Work out the finished part from the listing and answer in its coordinate system (mm). Face numbers are marked on the shaded views. A direction names the side the tool comes from. Give positions to 0.01 mm unless a question says otherwise; leave off trailing zeros. Loops run counter-clockwise (first coordinate to the right, second up) from the corner with the lowest first, then second, coordinate; pieces in that order, holes last. Notation, with made-up numbers: (39.25, 16) -> (71.25, 16) arc R22 cw to (71.25, 52) -> close; hole circle Ø9 at (19, -23). An arc over 180 degrees is marked (long way). Answer as CSV lines item,"result". Start each with the question number.
1. Find the intervals of material crossed by line 1 along X through (y, z) = (2.2, 8); line 2 along X through (y, z) = (4.35, 5); line 3 along Z through (x, y) = (31.5, 0.7), in increasing order.
2. Find section D-D, the plane z = -11. Give the vertices of the cut face in (x, y), and give its area (3 significant figures).
3. Find section C-C, the plane y = 2.9. Give the vertices of the cut face in (x, z) (1 decimal), and give its area (3 significant figures).
4. Determine the mould class of the marked faces 3, 4 and 5 for opening direction X: +X half, -X half, draft (parallel to the pull), parting line (faces both ways), or undercut.
5. A tool of negligible diameter and unlimited length cuts with its end or side. For the marked faces 1 and 2, from which of +Z, -Z, +X, -X, +Y, -Y can it reach the whole face along a straight path? Write none if from no direction.
6. Find section B-B, the plane z = -21. Give the vertices of the cut face in (x, y), and give its area (3 significant figures).
7. Flat-ended cylindrical pins translate along their axes: pin 1 Ø1 at (y, z) = (3, -8) entering from -X; pin 2 Ø1.5 at (x, y) = (-3, 3.5) entering from -Z; pin 3 Ø8 at (x, z) = (34.83, 4.17) entering from +Y; pin 4 Ø1.5 at (x, y) = (15.5, 3.5) entering from +Z. Find the tip coordinate at first contact, or state that the pin passes through.
8. Find section A-A, the plane x = 36. Give the vertices of the cut face in (y, z).
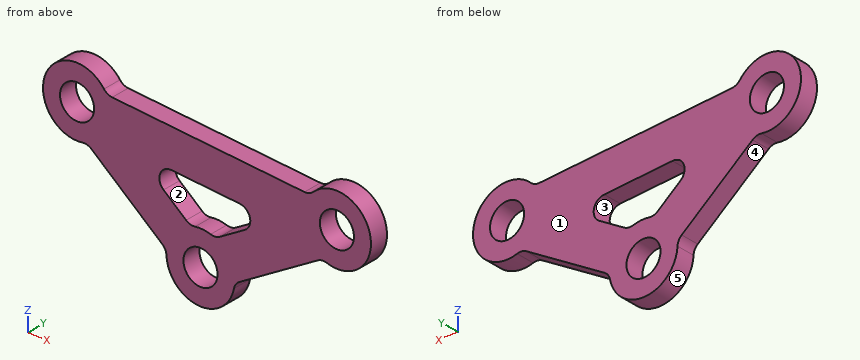
from build123d import *

# Parameters (mm, degrees)
SKETCH_1_R      = 4.5
EXTRUDE_1_DEPTH = 5


with BuildPart() as part:
    # 草图1 → 凸台-拉伸1 (new body)
    with BuildSketch(Plane(origin=(0, 0, 0), x_dir=(1, 0, 0), z_dir=(0, 1, 0))):
        with BuildLine():
            Line((-24.529804943, -13.414912777), (26.261252101, -9.790256419))
            ThreePointArc((26.261252101, -9.790256419), (27.501496461, -9.963799505), (28.562830813, -10.628549584))
            ThreePointArc((28.562830813, -10.628549584), (43.581244656, -6.254750357), (32.154801632, 4.427911945))
            ThreePointArc((32.154801632, 4.427911945), (30.907676626, 4.313883471), (29.722660532, 4.718926844))
            Line((29.722660532, 4.718926844), (9.037370221, 17.10767512))
            ThreePointArc((9.037370221, 17.10767512), (8.120961743, 17.961208234), (7.63285252, 19.114495996))
            ThreePointArc((7.63285252, 19.114495996), (-1.845653191, 26.39100116), (-10.194803688, 17.842241957))
            ThreePointArc((-10.194803688, 17.842241957), (-10.514193846, 16.631327756), (-11.300109489, 15.656309871))
            Line((-11.300109489, 15.656309871), (-30.016510781, 0.455696667))
            ThreePointArc((-30.016510781, 0.455696667), (-31.131999709, -0.113520099), (-32.382678895, -0.177745089))
            ThreePointArc((-32.382678895, -0.177745089), (-42.176335122, -12.374759959), (-26.689017586, -14.571546152))
            ThreePointArc((-26.689017586, -14.571546152), (-25.732836633, -13.762817978), (-24.529804943, -13.414912777))
        make_face()
        with Locations(Location((34.826919636, -4.166259648, 0), (0, 0, 270))):
            Circle(SKETCH_1_R, mode=Mode.SUBTRACT)
        with Locations(Location((-1.205005877, 17.413831728, 0), (0, 0, 270))):
            Circle(SKETCH_1_R, mode=Mode.SUBTRACT)
        with Locations(Location((-33.807302827, -9.064276845, 0), (0, 0, 270))):
            Circle(SKETCH_1_R, mode=Mode.SUBTRACT)
        with BuildLine():
            Line((-8.854823413, -2.270850546), (9.162609873, -0.985053244))
            ThreePointArc((9.162609873, -0.985053244), (11.867169109, 1.311172997), (10.490495867, 4.581045532))
            Line((10.490495867, 4.581045532), (3.899253226, 8.528645235))
            ThreePointArc((3.899253226, 8.528645235), (2.714237133, 8.933688608), (1.467112127, 8.819660134))
            ThreePointArc((1.467112127, 8.819660134), (-0.564358564, 8.436662295), (-2.62962981, 8.527299972))
            ThreePointArc((-2.62962981, 8.527299972), (-3.880308996, 8.463074982), (-4.995797924, 7.893858216))
            Line((-4.995797924, 7.893858216), (-10.959665987, 3.050274761))
            ThreePointArc((-10.959665987, 3.050274761), (-11.85804995, -0.381955107), (-8.854823413, -2.270850546))
        make_face(mode=Mode.SUBTRACT)
    extrude(amount=EXTRUDE_1_DEPTH)


solid = part.part
Resolved:
1,line 1,"x = -42.74 to -38.18, -29.43 to 32.47, 37.18 to 42.97"
1,line 2,"x = -41.84 to -35.74, -31.88 to 30.4, 39.25 to 43.79"
1,line 3,"z = -4.3 to 1.14, 7.2 to 12.53"
2,outline,"(-17.03, 0) -> (19.24, 0) -> (19.24, 5) -> (-17.03, 5) -> close"
2,area,"181 mm^2"
3,outline,"(-32.4, 0.2) arc R3 cw to (-30, -0.5) -> (-11.3, -15.7) arc R3 cw to (-10.2, -17.8) arc R9 ccw to (7.6, -19.1) arc R3 cw to (9, -17.1) -> (29.7, -4.7) arc R3 cw to (32.2, -4.4) arc R9 ccw (long way) to (28.6, 10.6) arc R3 cw to (26.3, 9.8) -> (-24.5, 13.4) arc R3 cw to (-26.7, 14.6) arc R9 ccw (long way) to start; hole circle Ø9 at (-33.8, 9.1); hole (-11, -3.1) -> (-5, -7.9) arc R3 ccw to (-2.6, -8.5) arc R9 cw to (1.5, -8.8) arc R3 ccw to (3.9, -8.5) -> (10.5, -4.6) arc R3 ccw to (9.2, 1) -> (-8.9, 2.3) arc R3 ccw to start; hole circle Ø9 at (-1.2, -17.4); hole circle Ø9 at (34.8, 4.2)"
3,area,"1,590 mm^2"
4,face 3,"undercut"
4,face 4,"-X half"
4,face 5,"parting line"
5,face 1,"+Z, -Z, +X, -X, +Y"
5,face 2,"+Y, -Y"
6,outline,"(-9.46, 0) -> (-3.92, 0) -> (-3.92, 5) -> (-9.46, 5) -> close; (1.51, 0) -> (7.05, 0) -> (7.05, 5) -> (1.51, 5) -> close"
6,area,"55.4 mm^2"
7,pin 1,"stops at x = -21.34"
7,pin 2,"stops at z = -26.35"
7,pin 3,"passes through"
7,pin 4,"stops at z = 10.61"
8,outline,"(0, -4.76) -> (5, -4.76) -> (5, -0.18) -> (0, -0.18) -> close; (0, 8.51) -> (5, 8.51) -> (5, 13.09) -> (0, 13.09) -> close"
